Geometry: final body of the model. Coordinates: model frame, mm. A direction names the side the tool comes from. Round coordinates to 2 decimals unless told otherwise and drop trailing zeros. Loops run counter-clockwise (first coordinate to the right, second up) from the corner with the lowest first, then second, coordinate; pieces in that order, holes last. Notation, with made-up numbers: (-24.75, -21.75) -> (-2.75, -21.75) arc R14 cw to (-2.75, -2.75) -> close; hole circle Ø8 at (83, 52.25). An arc over 180 degrees is marked (long way). Answer in a Markdown table with one row per item.
```python
from build123d import *

# Parameters (mm, degrees)
SKETCH1_R           = 32.5
SKETCH1_R_2         = 20.625
BOSS_EXTRUDE1_DEPTH = 17
BOSS_EXTRUDE2_START = 24
SKETCH2_W           = 45
SKETCH2_H           = 24
BOSS_EXTRUDE2_DEPTH = 72
SKETCH4_R           = 5
CUT_EXTRUDE1_DEPTH  = 103.767942472
SKETCH7_R           = 5
BOSS_EXTRUDE3_DEPTH = 25
BOSS_EXTRUDE4_REACH = 204.691
SKETCH8_R           = 22
SKETCH8_R_2         = 11.1
BOSS_EXTRUDE5_REACH = 183.31
SKETCH10_R          = 14
SKETCH10_R_2        = 5
SKETCH14_R          = 5
CUT_EXTRUDE3_DEPTH  = 34
CUT_EXTRUDE4_REACH  = 175.842


with BuildPart() as part:
    # Sketch1 → Boss-Extrude1 (new, symmetric)
    with BuildSketch(Plane.XY):
        Circle(SKETCH1_R)
        Circle(SKETCH1_R_2, mode=Mode.SUBTRACT)
    extrude(amount=BOSS_EXTRUDE1_DEPTH, both=True)

    # Sketch2 → Boss-Extrude2 (add)
    with BuildSketch(Plane(origin=(0, 0, 0), x_dir=(1, 0, 0), z_dir=(0, 1, 0)).offset(BOSS_EXTRUDE2_START)):
        Rectangle(SKETCH2_W, SKETCH2_H)
    extrude(amount=BOSS_EXTRUDE2_DEPTH)

    # Sketch4 → Cut-Extrude1 (cut, through all)
    with BuildSketch(Plane(origin=(0, 0, 0), x_dir=(0, 0, -1), z_dir=(1, 0, 0))):
        with Locations(Location((0, 0, 0), (0, 0, 180))):
            Circle(SKETCH4_R)
    extrude(amount=CUT_EXTRUDE1_DEPTH, mode=Mode.SUBTRACT)

    # Sketch7 → Boss-Extrude3 (add, symmetric)
    with BuildSketch(Plane.XY):
        with BuildLine():
            Line((-13, 64), (13, 64))
            Line((13, 64), (22.792288735, 85.728117298))
            ThreePointArc((22.792288735, 85.728117298), (24.050431537, 102.824715589), (14, 116.712315177))
            Line((14, 116.712315177), (14, 140))
            ThreePointArc((14, 140), (0, 154), (-14, 140))
            Line((-14, 140), (-14, 116.712315177))
            ThreePointArc((-14, 116.712315177), (-24.050431537, 102.824715589), (-22.792288735, 85.728117298))
            Line((-22.792288735, 85.728117298), (-13, 64))
        make_face()
        with Locations((0, 140)):
            Circle(SKETCH7_R, mode=Mode.SUBTRACT)
        with BuildLine():
            Line((-6, 73.61), (6, 73.61))
            Line((6, 73.61), (6, 79.613954107))
            ThreePointArc((6, 79.613954107), (0, 113.45), (-6, 79.613954107))
            Line((-6, 79.613954107), (-6, 73.61))
        make_face(mode=Mode.SUBTRACT)
    extrude(amount=BOSS_EXTRUDE3_DEPTH, both=True)

    # Sketch8 → Boss-Extrude4 (add, up to next)
    with BuildSketch(Plane(origin=(0, 166, 0), x_dir=(1, 0, 0), z_dir=(0, 1, 0)), mode=Mode.PRIVATE) as boss_extrude4_sk1:
        with Locations(Location((0, 0, 0), (0, 0, 270))):
            Circle(SKETCH8_R)
        with Locations(Location((0, 0, 0), (0, 0, 270))):
            Circle(SKETCH8_R_2, mode=Mode.SUBTRACT)
    boss_extrude4_tool1 = extrude(boss_extrude4_sk1.sketch, amount=-BOSS_EXTRUDE4_REACH, mode=Mode.PRIVATE) - part.part
    add(boss_extrude4_tool1.solids().sort_by_distance((0, 166, -21.377746))[0])

    # Sketch10 → Boss-Extrude5 (add, up to next)
    with BuildSketch(Plane(origin=(36, 0, 0), x_dir=(0, 0, -1), z_dir=(1, 0, 0)), mode=Mode.PRIVATE) as boss_extrude5_sk1:
        with Locations((0, 96)):
            Circle(SKETCH10_R)
        with Locations((0, 96)):
            Circle(SKETCH10_R_2, mode=Mode.SUBTRACT)
    boss_extrude5_tool1 = extrude(boss_extrude5_sk1.sketch, amount=-BOSS_EXTRUDE5_REACH, mode=Mode.PRIVATE) - part.part
    add(boss_extrude5_tool1.solids().sort_by_distance((36, 96, 13.60402))[0])

    # Sketch14 → Cut-Extrude3 (cut)
    with BuildSketch(Plane(origin=(36, 0, 0), x_dir=(0, 0, -1), z_dir=(1, 0, 0))):
        with Locations((0, 96)):
            Circle(SKETCH14_R)
    extrude(amount=-CUT_EXTRUDE3_DEPTH, mode=Mode.SUBTRACT)

    # Sketch15 → Cut-Extrude4 (cut, up to next)
    with BuildSketch(Plane.XY.offset(12), mode=Mode.PRIVATE) as cut_extrude4_sk1:
        with BuildLine():
            Line((6, 73.61), (6, 79.613954107))
            ThreePointArc((6, 79.613954107), (14.303889331, 86.00493872), (17.45, 96))
            Line((17.45, 96), (-17.45, 96))
            ThreePointArc((-17.45, 96), (-14.303889331, 86.00493872), (-6, 79.613954107))
            Line((-6, 79.613954107), (-6, 73.61))
            Line((-6, 73.61), (6, 73.61))
        make_face()
    cut_extrude4_tool1 = extrude(cut_extrude4_sk1.sketch, amount=-CUT_EXTRUDE4_REACH, mode=Mode.PRIVATE) & part.part
    add(cut_extrude4_tool1.solids().sort_by_distance((0, 87.149335, 12))[0], mode=Mode.SUBTRACT)


solid = part.part
```
Item 1: Draft query along Y for faces 5 (the face through (5.2, 166, -10.1)), 6 (the face through (-4.471, -20.135, -0.238)), 7 (the face through (14, 128, -21)). Return one class per face: pulls with the +Y half, pulls with the -Y half, needs draft (parallel to the pull), parting line crosses it, or undercut.
Answer:
| item | result |
|---|---|
| face 5 | pulls with the +Y half |
| face 6 | undercut |
| face 7 | needs draft |
Item 2: Line query: probe 1 along Y at (x, z) = (0, 13) (3 decimals); probe 2 along Y at (x, z) = (0, -6) (3 decimals); probe 3 along Y at (x, z) = (-3, 5). Output: solid intervals per line, ascending. Write a range as [from, to].
Answer:
| item | result |
|---|---|
| probe 1 | y = [-32.5, -20.625], [20.625, 32.5], [64, 73.61], [113.45, 135], [145, 166] |
| probe 2 | y = [-32.5, -20.625], [20.625, 73.61], [113.45, 135], [145, 154] |
| probe 3 | y = [-32.36, -20.41], [20.41, 73.61], [113.19, 136], [144, 153.67] |
Item 3: Reachability of faces 1 (the face through (14, 128, 21)), 2 (the face through (0, 154, -23)), 3 (the face through (-14, 129, 21)), 4 (the face through (30.41, 109.88, 1.82)) from +Z, -Z, +X, -X, +Y, -Y: full face, straight path, thin tool, end or side. Return the list, or none.
Answer:
| item | result |
|---|---|
| face 1 | +Z, +X, +Y |
| face 2 | -Z, +Y |
| face 3 | +Z, -X, +Y |
| face 4 | +X |
Item 4: Cut plane A-A (x = 0). Count the separate pieces of the cut face and the enclosed holes in it, then the cut area to 3 significant figures.
Answer:
| item | result |
|---|---|
| separate pieces | 4 |
| enclosed holes | 0 |
| area | 3,830 mm² |
Item 5: Pin query (flat end, axial travel): pin 1 Ø6 at (x, y) = (28.5, -0.5) entering from -Z; pin 2 Ø13 at (y, z) = (96, 0) entering from +X; pin 3 Ø8 at (y, z) = (7, 18) entering from +X; pin 4 Ø1 at (y, z) = (123.5, -7) entering from +X. Return the tip coordinate at first contact, or that it passes through.
Answer:
| item | result |
|---|---|
| pin 1 | stops at z = -17 |
| pin 2 | stops at x = 36 |
| pin 3 | stops at x = 32.35 |
| pin 4 | stops at x = 21.02 |
Item 6: Cut plane B-B (y = 0). Output: boundary loops of the cut face in (x, z) (3 decimals), then the cut area to 3 significant figures.
Answer:
| item | result |
|---|---|
| outline | (-32.5, -17) -> (-20.625, -17) -> (-20.625, 17) -> (-32.5, 17) -> close; (20.625, -17) -> (32.5, -17) -> (32.5, -5) -> (20.625, -5) -> close; (20.625, 5) -> (32.5, 5) -> (32.5, 17) -> (20.625, 17) -> close |
| area | 689 mm² |
Item 7: Cut plane C-C (x = 29). Output: boundary loops of the cut face in (y, z), then the cut area to 3 significant figures.
Answer:
| item | result |
|---|---|
| outline | (-14.67, -17) -> (14.67, -17) -> (14.67, 17) -> (-14.67, 17) -> close; circle Ø28 at (96, 0); hole circle Ø10 at (0, 0); hole circle Ø10 at (96, 0) |
| area | 1,460 mm² |
